Check sheet for the drawn part. Datum: minimum x, y, z corner. Units: mm. A direction names the side the tool comes from. Round coordinates to 2 decimals unless told otherwise and drop trailing zeros. Write each loop counter-clockwise with the first axis right and the second up, starting at its lowest first coordinate (ties: lowest second). Pieces come first, ordered by that corner, then holes. Notation, with made-up numbers: (12, 47) -> (38, 47) arc R11 cw to (38, 63) -> close; hole circle Ø8 at (-22, 22). An arc over 180 degrees is marked (long way). One line per item, written item: value. Start each with the question number.
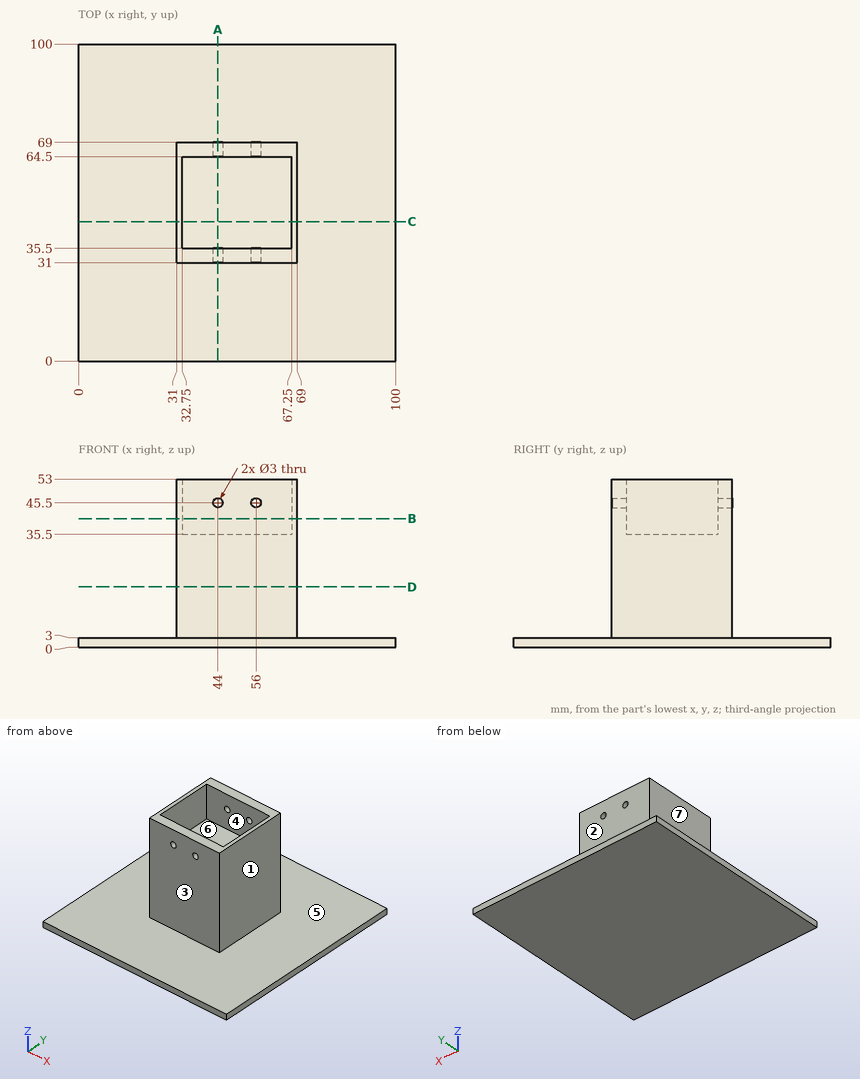
1. Cross-section at A-A (x = 44). Record the cut outline in (y, z).
2. Depth check by flat-ended pin: pin 1 Ø14 at (x, z) = (43, 46.5) entering from +Y; pin 2 Ø2.5 at (x, z) = (44, 45.5) entering from +Y; pin 3 Ø10 at (x, y) = (40.5, 78) entering from -Z; pin 4 Ø14 at (x, z) = (52.5, 48) entering from -Y. Enter the tip coordinate at first touch or a pass-through.
3. Release check for a two-part mould opening along X. For the marked faces 4, 5, 6 and 7 record: +X half, -X half, draft (parallel to the pull), parting line (faces both ways), or undercut.
4. Cross-section at D-D (z = 19). Record the cut outline in (x, y), plus the area to 3 significant figures.
5. Access from +Z, -Z, +X, -X, +Y, -Y to the whole of each face (thin tool, end or side, straight path). Record for the marked faces 1, 2 and 3.
6. Material ranges on probe 1 along X at (y, z) = (65.5, 45.5); probe 2 along Y at (x, z) = (64.5, 39); probe 3 along X at (y, z) = (66, 45), recorded low to high.
7. Cross-section at B-B (z = 40.5). Record the cut outline in (x, y).
8. Cross-section at C-C (y = 44). Record the cut outline in (x, z), plus the area to 3 significant figures.
Working result:
1. outline: (0, 0) -> (100, 0) -> (100, 3) -> (69, 3) -> (69, 44) -> (64.5, 44) -> (64.5, 35.5) -> (35.5, 35.5) -> (35.5, 44) -> (31, 44) -> (31, 3) -> (0, 3) -> close; (31, 47) -> (35.5, 47) -> (35.5, 53) -> (31, 53) -> close; (64.5, 47) -> (69, 47) -> (69, 53) -> (64.5, 53) -> close
2. pin 1: stops at y = 69
2. pin 2: passes through
2. pin 3: stops at z = 0
2. pin 4: stops at y = 31
3. face 4: undercut
3. face 5: draft
3. face 6: undercut
3. face 7: -X half
4. outline: (31, 31) -> (69, 31) -> (69, 69) -> (31, 69) -> close
4. area: 1,440 mm^2
5. face 1: +Z, +X, +Y, -Y
5. face 2: +Z, +X, -X, +Y
5. face 3: +Z, +X, -X, -Y
6. probe 1: x = 31 to 42.5, 45.5 to 54.5, 57.5 to 69
6. probe 2: y = 31 to 35.5, 64.5 to 69
6. probe 3: x = 31 to 42.59, 45.41 to 54.59, 57.41 to 69
7. outline: (31, 31) -> (69, 31) -> (69, 69) -> (31, 69) -> close; hole (32.75, 35.5) -> (67.25, 35.5) -> (67.25, 64.5) -> (32.75, 64.5) -> close
8. outline: (0, 0) -> (100, 0) -> (100, 3) -> (69, 3) -> (69, 53) -> (67.25, 53) -> (67.25, 35.5) -> (32.75, 35.5) -> (32.75, 53) -> (31, 53) -> (31, 3) -> (0, 3) -> close
8. area: 1,600 mm^2
